```python
from build123d import *

# Parameters (mm, degrees)
BOSS_EXTRUDE1_DEPTH = 60
CUT_EXTRUDE1_DEPTH  = 60


with BuildPart() as part:
    # Sketch1 → Boss-Extrude1 (new body)
    with BuildSketch(Plane.XY):
        with BuildLine():
            Line((-30, 50.32677643), (-30, 10.32677643))
            Line((-30, 10.32677643), (-15, 10.32677643))
            Line((-15, 10.32677643), (-15, 20.32677643))
            Line((-15, 20.32677643), (15, 20.32677643))
            Line((15, 20.32677643), (15, 10.32677643))
            Line((15, 10.32677643), (80, 10.32677643))
            Line((80, 10.32677643), (80, 20.32677643))
            Line((80, 20.32677643), (30, 20.32677643))
            Line((30, 20.32677643), (30, 50.32677643))
            Line((30, 50.32677643), (15, 50.32677643))
            ThreePointArc((15, 50.32677643), (0, 35.32677643), (-15, 50.32677643))
            Line((-15, 50.32677643), (-30, 50.32677643))
        make_face()
    extrude(amount=BOSS_EXTRUDE1_DEPTH)

    # Sketch2 → Cut-Extrude1 (cut)
    with BuildSketch(Plane(origin=(0, 20.32677643, 0), x_dir=(1, 0, 0), z_dir=(0, 1, 0))):
        with BuildLine():
            Line((80, -15), (80, -45))
            Line((80, -45), (60, -45))
            ThreePointArc((60, -45), (45, -30), (60, -15))
            Line((60, -15), (80, -15))
        make_face()
    extrude(amount=-CUT_EXTRUDE1_DEPTH, mode=Mode.SUBTRACT)


solid = part.part
```
The model under review builds one solid part; all positions refer to its coordinate system, in mm. A direction names the side the tool comes from. Round coordinates to 2 decimals unless told otherwise and drop trailing zeros. Loops run counter-clockwise (first coordinate to the right, second up) from the corner with the lowest first, then second, coordinate; pieces in that order, holes last. Notation, with made-up numbers: (33.25, 44.5) -> (88.25, 44.5) arc R24 cw to (88.25, 56.5) -> close; hole circle Ø8 at (72.5, 55.25). An arc over 180 degrees is marked (long way). Answer as a JSON object with one key per item and string values. Group by question number.
1) For pin 1 Ø8 at (y, z) = (16.5, 39.5) entering from +X; pin 2 Ø10 at (x, z) = (8, 42.5) entering from +Y; pin 3 Ø24 at (y, z) = (41, 37.5) entering from +X, all flat-tipped, find the tip position at first contact; note any pin that passes through.
2) We need section C-C on z = 56.5. Write out the cut boundary in (x, y), then the cut area to 3 significant figures.
3) We need section B-B on y = 19. Write out the cut boundary in (x, z), then the cut area to 3 significant figures.
4) We need section D-D on x = 0. Write out the cut boundary in (y, z), then the cut area to 3 significant figures.
5) For line 1 (X direction, y = 16, z = 29.5); line 2 (Y direction, x = 39.5, z = 25.5); line 3 (X direction, y = 43, z = 18.5), list the stretches that pass through material, from the lowest coordinate up. Write a range as [from, to].
6) We need section A-A on x = 71. Write out the cut boundary in (y, z).
7) For faces 1 (the face through (70, 15, 15)), 2 (the face through (15, 15, 30)), 3 (the face through (44, 20.327, 30)), list the 3-axis set-ups (+Z, -Z, +X, -X, +Y, -Y) from which the entire face can be reached by the end or side of a thin tool; tool diameter is ignored.
8) Mouldability with a two-part tool opening along Z and no side actions: class faces 4 (the face through (12, 26, 60)), 5 (the face through (45, 15, 30)), 6 (the face through (70, 15, 45)), 7 (the face through (40, 10.327, 30)) as released by +Z, released by -Z, zero draft, split by the parting line, or undercut.
Result set:
{
 "1": {"pin 1": "x = 53.46", "pin 2": "y = 42.84", "pin 3": "x = 30"},
 "2": {"outline": "(-30, 10.33) -> (-15, 10.33) -> (-15, 20.33) -> (15, 20.33) -> (15, 10.33) -> (80, 10.33) -> (80, 20.33) -> (30, 20.33) -> (30, 50.33) -> (15, 50.33) arc R15 cw to (-15, 50.33) -> (-30, 50.33) -> close", "area": "2,250 mm²"},
 "3": {"outline": "(-30, 0) -> (-15, 0) -> (-15, 60) -> (-30, 60) -> close; (15, 0) -> (80, 0) -> (80, 15) -> (60, 15) arc R15 cw to (60, 45) -> (80, 45) -> (80, 60) -> (15, 60) -> close", "area": "3,850 mm²"},
 "4": {"outline": "(20.33, 0) -> (35.33, 0) -> (35.33, 60) -> (20.33, 60) -> close", "area": "900 mm²"},
 "5": {"line 1": "[-30, -15], [15, 45.01]", "line 2": "[10.33, 20.33]", "line 3": "[-30, -13.09], [13.09, 30]"},
 "6": {"outline": "(10.33, 0) -> (20.33, 0) -> (20.33, 15) -> (10.33, 15) -> close; (10.33, 45) -> (20.33, 45) -> (20.33, 60) -> (10.33, 60) -> close"},
 "7": {"face 1": "+X, +Y, -Y", "face 2": "+Z, -Z, -Y", "face 3": "+Z, -Z, +X, +Y"},
 "8": {"face 4": "released by +Z", "face 5": "undercut", "face 6": "undercut", "face 7": "zero draft"}
}
